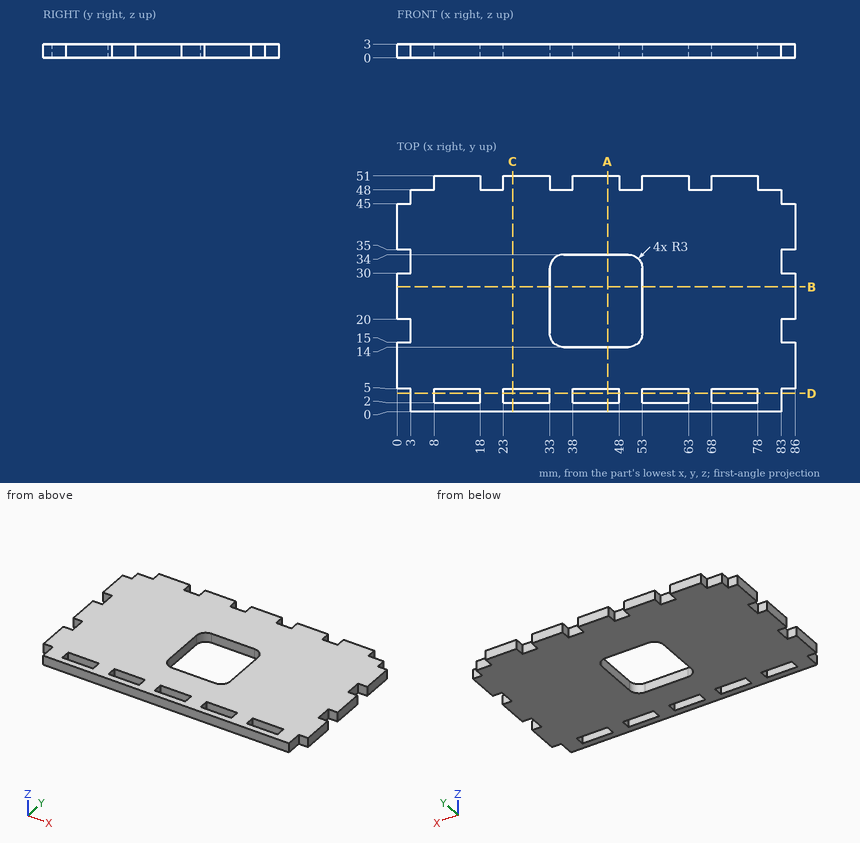
Can you work these out from the drawing? Everything is in mm from the part's minimum corner. Round coordinates to 2 decimals unless told otherwise and drop trailing zeros. Order: outer loops, then holes, each group sorted by start corner. A loop starts at its lowest first (then second) coordinate and runs counter-clockwise, first axis right, second up. Notation, with made-up numbers: (-34, 9.5) - (-9, 9.5) arc R17 cw to (-9, 32.5) - close; hole circle Ø4 at (47, 82). An arc over 180 degrees is marked (long way). Answer in a Markdown table with one row per item.
(1) Suppose I cut it at A-A, the plane x = 45.5. Please give me the cut outline in (y, z).
From the geometry:
| item | result |
|---|---|
| outline | (0, 0) - (2, 0) - (2, 3) - (0, 3) - close; (5, 0) - (14, 0) - (14, 3) - (5, 3) - close; (34, 0) - (51, 0) - (51, 3) - (34, 3) - close |
(2) For P1, Ø0.9, axis at y = 3.5, z = 1.5, coming from the -X side; P2, Ø0.9, axis at y = 50, z = 2, coming from the +X side; P3, Ø1.5, axis at x = 42.5, z = 2.5, coming from the -Y side; P4, Ø1.5, axis at x = 1, z = 1.5, coming from the +Y side, each with a flat end and sliding along its axis, tell me the tip position at first contact or that it passes through.
From the geometry:
| item | result |
|---|---|
| P1 | stops at x = 3 |
| P2 | stops at x = 78 |
| P3 | stops at y = 0 |
| P4 | stops at y = 45 |
(3) Please list where these lines run through material, in increasing order: L1, parallel to X at y = 3, z = 0.8; L2, parallel to Y at x = 76.5, z = 0.1; L3, parallel to X at y = 20.5, z = 1.7. Write a range as from..to.
From the geometry:
| item | result |
|---|---|
| L1 | x = 3..8, 18..23, 33..38, 48..53, 63..68, 78..83 |
| L2 | y = 0..2, 5..51 |
| L3 | x = 0..33, 53..86 |
(4) Suppose I cut it at B-B, the plane y = 27. Please give me the cut outline in (x, z).
From the geometry:
| item | result |
|---|---|
| outline | (0, 0) - (33, 0) - (33, 3) - (0, 3) - close; (53, 0) - (86, 0) - (86, 3) - (53, 3) - close |
(5) Suppose I cut it at C-C, the plane x = 25. Please give me the cut outline in (y, z).
From the geometry:
| item | result |
|---|---|
| outline | (0, 0) - (2, 0) - (2, 3) - (0, 3) - close; (5, 0) - (51, 0) - (51, 3) - (5, 3) - close |
(6) Suppose I cut it at D-D, the plane y = 4. Please give me the cut outline in (x, z), plus the area to 3 significant figures.
From the geometry:
| item | result |
|---|---|
| outline | (3, 0) - (8, 0) - (8, 3) - (3, 3) - close; (18, 0) - (23, 0) - (23, 3) - (18, 3) - close; (33, 0) - (38, 0) - (38, 3) - (33, 3) - close; (48, 0) - (53, 0) - (53, 3) - (48, 3) - close; (63, 0) - (68, 0) - (68, 3) - (63, 3) - close; (78, 0) - (83, 0) - (83, 3) - (78, 3) - close |
| area | 90.0 mm2 |
